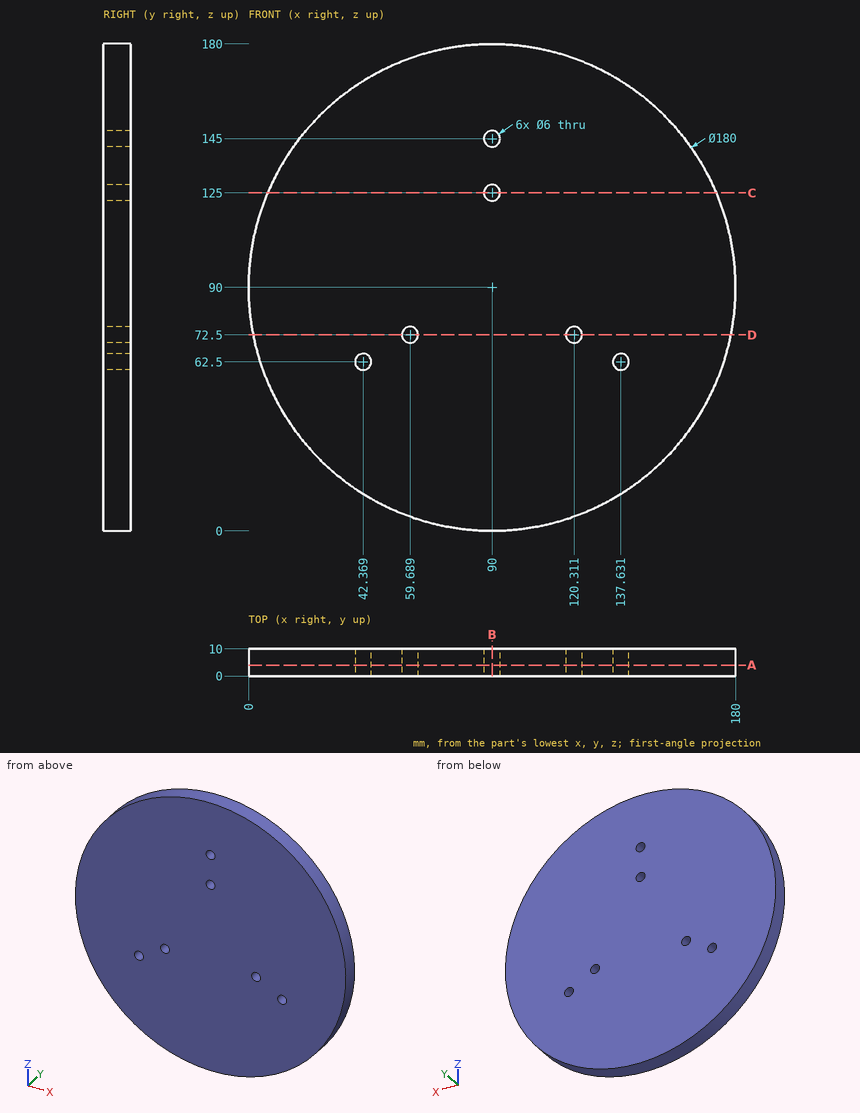
Design review of the part shown in the three views and the two pictorial views. Dimensions are in mm from the part's minimum x, y and z. Coordinates: 2 decimals unless noted, no trailing zeros. Loops run counter-clockwise (first coordinate to the right, second up) from the corner with the lowest first, then second, coordinate; pieces in that order, holes last.
(1) Wall thickness on L1, parallel to X at y = 4, z = 145; L2, parallel to Z at x = 43, y = 8; L3, parallel to X at y = 3.5, z = 111.5 (1 decimal): over which ranges is each line inside the solid? List them lowest first.
Determined:
L1: x = 18.76 to 87, 93 to 161.24
L2: z = 13.25 to 59.57, 65.43 to 166.75
L3: x = 2.6 to 177.4
(2) Consider section B-B, the plane x = 90. Give the boundary of the cut face in (y, z).
Determined:
outline: (0, 0) - (10, 0) - (10, 122) - (0, 122) - close; (0, 128) - (10, 128) - (10, 142) - (0, 142) - close; (0, 148) - (10, 148) - (10, 180) - (0, 180) - close
(3) Consider section C-C, the plane z = 125. Give the boundary of the cut face in (x, y) (1 decimal).
Determined:
outline: (7.1, 0) - (87, 0) - (87, 10) - (7.1, 10) - close; (93, 0) - (172.9, 0) - (172.9, 10) - (93, 10) - close
(4) Insertion check: P1, Ø3, axis at x = 104.5, y = 1.5, coming from the -Z side; P2, Ø5, axis at x = 103.5, y = 4, coming from the +Z side (1 decimal); P3, Ø6, axis at x = 64, y = 2.5, coming from the -Z side. Each pin has a flat end and moves straight along its axis. Give the tip position at first contact, or say it passes through.
Determined:
P1: stops at z = 0.94
P2: stops at z = 179.3
P3: stops at z = 2.99
(5) Consider section A-A, the plane y = 4. Give the boundary of the cut face in (x, z).
Determined:
outline: circle Ø180 at (90, 90); hole circle Ø6 at (42.37, 62.5); hole circle Ø6 at (59.69, 72.5); hole circle Ø6 at (90, 125); hole circle Ø6 at (90, 145); hole circle Ø6 at (120.31, 72.5); hole circle Ø6 at (137.63, 62.5)
(6) Consider section D-D, the plane z = 72.5. Give the boundary of the cut face in (x, y), plus the area to 3 significant figures.
Determined:
outline: (1.72, 0) - (56.69, 0) - (56.69, 10) - (1.72, 10) - close; (62.69, 0) - (117.31, 0) - (117.31, 10) - (62.69, 10) - close; (123.31, 0) - (178.28, 0) - (178.28, 10) - (123.31, 10) - close
area: 1,650 mm2
